Design review of the part built by this model. Coordinates are the model's own, in mm. A direction names the side the tool comes from. Coordinates: 2 decimals unless noted, no trailing zeros. Write each loop counter-clockwise with the first axis right and the second up, starting at its lowest first coordinate (ties: lowest second). Pieces come first, ordered by that corner, then holes. Notation, with made-up numbers: (30.25, 16) -> (86.25, 16) arc R19 cw to (86.25, 44) -> close; hole circle Ø1 at (25, 25). An arc over 180 degrees is marked (long way). One line per question, with ' | ' between items. Start each with the question number.
Q1. Wall thickness on probe 1 along X at (y, z) = (-47, 17); probe 2 along Z at (x, y) = (-128, -32); probe 3 along Z at (x, y) = (0, -3.1): over which ranges is each line inside the solid? List them lowest first.
Q2. Add section A-A on x = 0. State the section outline as (y, z) points.
Q3. For faces 4 (the flat face through (-128.25, -33, -1)), 5 (the cylindrical face through (23.846, -2.465, -7.509)), list the 3-axis set-ups (+Z, -Z, +X, -X, +Y, -Y) from which the entire face can be reached by the end or side of a thin tool; tool diameter is ignored.
Q4. For P1, Ø1.2, axis at x = -128.25, z = 64.25, coming from the -Y side, flat-tipped, find the tip position at first contact; note if it passes through.
Q5. Add section D-D on x = -42. State the section outline as (y, z) points, and give its area (3 significant figures).
Q6. Add section C-C on y = -40.5. State the section outline as (x, z) points.
Q7. Draft analysis for pull direction X (two halves, no side actions). For faces 1 (the flat face through (-133, -30, -1)), 2 (the flat face through (128.25, -33, -1)), 3 (the flat face through (-40, -60, 67)), state which applies: pulls with the +X half, pulls with the -X half, needs draft (parallel to the pull), parting line crosses it, or undercut.
Q8. Add section B-B on z = 0. State the section outline as (x, y) points, and give its area (3 significant figures).
from build123d import *

# Parameters (mm, degrees)
SKETCH_W        = 266
SKETCH_H        = 138
PAD_DEPTH       = 60
SKETCH001_W     = 256.5
SKETCH001_H     = 128.5
POCKET_DEPTH    = 55
FILLET_R        = 2
SKETCH002_R     = 25
POCKET001_DEPTH = 60.001
SKETCH003_R     = 1
POCKET002_DEPTH = 55


with BuildPart() as part:
    # Sketch → Pad (new body)
    with BuildSketch(Plane.XZ):
        Rectangle(SKETCH_W, SKETCH_H)
    extrude(amount=PAD_DEPTH)

    # Sketch001 (on Face6 of Pad) → Pocket (cut)
    with BuildSketch(Plane.XZ.offset(60)):
        Rectangle(SKETCH001_W, SKETCH001_H)
    extrude(amount=-POCKET_DEPTH, mode=Mode.SUBTRACT)

    # Fillet
    fillet_edges = [part.edges().sort_by_distance(p)[0] for p in [
        (-133, -30, 69),
        (133, -30, 69),
        (-133, -30, -69),
        (133, -30, -69),
    ]]
    fillet(fillet_edges, radius=FILLET_R)

    # Sketch002 (on Face2 of Fillet) → Pocket001 (cut, through all)
    with BuildSketch(Plane(origin=(0, 0, 0), x_dir=(1, 0, 0), z_dir=(0, 1, 0))):
        Circle(SKETCH002_R)
    extrude(amount=-POCKET001_DEPTH, mode=Mode.SUBTRACT)

    # Sketch003 (on Face5 of Pocket) → Pocket002 (cut)
    with BuildSketch(Plane.XZ.offset(60)):
        with Locations((-128.25, 64.25)):
            Circle(SKETCH003_R)
        with Locations((128.25, 64.25)):
            Circle(SKETCH003_R)
        with Locations((128.25, -64.25)):
            Circle(SKETCH003_R)
        with Locations((-128.25, -64.25)):
            Circle(SKETCH003_R)
    extrude(amount=-POCKET002_DEPTH, mode=Mode.SUBTRACT)


solid = part.part
Output values:
1) probe 1: x = -133 to -128.25, 128.25 to 133 | probe 2: z = -69 to -65.22, 65.22 to 69 | probe 3: z = -69 to -25, 25 to 69
2) outline: (-60, -69) -> (0, -69) -> (0, -25) -> (-5, -25) -> (-5, -64.25) -> (-60, -64.25) -> close; (-60, 64.25) -> (-5, 64.25) -> (-5, 25) -> (0, 25) -> (0, 69) -> (-60, 69) -> close
3) face 4: -Y | face 5: +Y, -Y
4) P1: stops at y = -5
5) outline: (-60, -69) -> (0, -69) -> (0, 69) -> (-60, 69) -> (-60, 64.25) -> (-5, 64.25) -> (-5, -64.25) -> (-60, -64.25) -> close | area: 1,210 mm2
6) outline: (-133, -67) arc R2 ccw to (-131, -69) -> (131, -69) arc R2 ccw to (133, -67) -> (133, 67) arc R2 ccw to (131, 69) -> (-131, 69) arc R2 ccw to (-133, 67) -> close; hole (-128.25, -63.25) arc R1 ccw (long way) to (-127.25, -64.25) -> (127.25, -64.25) arc R1 ccw (long way) to (128.25, -63.25) -> (128.25, 63.25) arc R1 ccw (long way) to (127.25, 64.25) -> (-127.25, 64.25) arc R1 ccw (long way) to (-128.25, 63.25) -> close
7) face 1: pulls with the -X half | face 2: undercut | face 3: needs draft
8) outline: (-133, -60) -> (-128.25, -60) -> (-128.25, -5) -> (-25, -5) -> (-25, 0) -> (-133, 0) -> close; (25, -5) -> (128.25, -5) -> (128.25, -60) -> (133, -60) -> (133, 0) -> (25, 0) -> close | area: 1,600 mm2
